```python
from build123d import *

# Parameters (mm, degrees)
F0_R     = 1.5
F1_DEPTH = 17
F2_DEPTH = 2
F3_R     = 5


with BuildPart() as f1:
    # F0 (on Top) → F1 (new body)
    with BuildSketch(Plane.XY):
        with BuildLine():
            ThreePointArc((21.4336734694, 1.6874956615), (21.4834119682, 0.8443993155), (21.5, 0))
            ThreePointArc((21.5, 0), (21.4834119682, -0.8443993155), (21.4336734694, -1.6874956615))
            ThreePointArc((21.4336734694, -1.6874956615), (22.0184319463, -2.4681612579), (22.7959183673, -3.0571401324))
            ThreePointArc((22.7959183673, -3.0571401324), (22.9489228772, -1.531972185), (23, 0))
            ThreePointArc((23, 0), (22.9489228772, 1.531972185), (22.7959183673, 3.0571401324))
            ThreePointArc((22.7959183673, 3.0571401324), (22.0184319463, 2.4681612579), (21.4336734694, 1.6874956615))
        make_face()
        with BuildLine():
            ThreePointArc((-21.4336734694, 1.6874956615), (0, 21.5), (21.4336734694, 1.6874956615))
            ThreePointArc((21.4336734694, 1.6874956615), (22.0184319463, 2.4681612579), (22.7959183673, 3.0571401324))
            ThreePointArc((22.7959183673, 3.0571401324), (0, 23), (-22.7959183673, 3.0571401324))
            ThreePointArc((-22.7959183673, 3.0571401324), (-22.0184319463, 2.4681612579), (-21.4336734694, 1.6874956615))
        make_face()
        with BuildLine():
            ThreePointArc((22.7959183673, -3.0571401324), (22.0184319463, -2.4681612579), (21.4336734694, -1.6874956615))
            ThreePointArc((21.4336734694, -1.6874956615), (0, -21.5), (-21.4336734694, -1.6874956615))
            ThreePointArc((-21.4336734694, -1.6874956615), (-22.0184319463, -2.4681612579), (-22.7959183673, -3.0571401324))
            ThreePointArc((-22.7959183673, -3.0571401324), (0, -23), (22.7959183673, -3.0571401324))
        make_face()
        with BuildLine():
            ThreePointArc((-21.4336734694, -1.6874956615), (-21.5, 0), (-21.4336734694, 1.6874956615))
            ThreePointArc((-21.4336734694, 1.6874956615), (-22.0184319463, 2.4681612579), (-22.7959183673, 3.0571401324))
            ThreePointArc((-22.7959183673, 3.0571401324), (-22.9489228772, 1.531972185), (-23, 0))
            ThreePointArc((-23, 0), (-22.9489228772, -1.531972185), (-22.7959183673, -3.0571401324))
            ThreePointArc((-22.7959183673, -3.0571401324), (-22.0184319463, -2.4681612579), (-21.4336734694, -1.6874956615))
        make_face()
        with BuildLine():
            ThreePointArc((28, 0), (26.2728105209, 3.0178043106), (22.7959183673, 3.0571401324))
            ThreePointArc((22.7959183673, 3.0571401324), (22.9489228772, 1.531972185), (23, 0))
            ThreePointArc((23, 0), (22.9489228772, -1.531972185), (22.7959183673, -3.0571401324))
            ThreePointArc((22.7959183673, -3.0571401324), (26.2728105209, -3.0178043106), (28, 0))
        make_face()
        with BuildLine():
            ThreePointArc((26, 0), (24.5, -1.5), (23, 0))
            ThreePointArc((23, 0), (24.5, 1.5), (26, 0))
        make_face(mode=Mode.SUBTRACT)
        with BuildLine():
            ThreePointArc((-23, 0), (-22.9489228772, 1.531972185), (-22.7959183673, 3.0571401324))
            ThreePointArc((-22.7959183673, 3.0571401324), (-28, 0), (-22.7959183673, -3.0571401324))
            ThreePointArc((-22.7959183673, -3.0571401324), (-22.9489228772, -1.531972185), (-23, 0))
        make_face()
        with Locations((-24.5, 0)):
            Circle(F0_R, mode=Mode.SUBTRACT)
    extrude(amount=F1_DEPTH)

    # F0 (on Top) → F2 (join)
    with BuildSketch(Plane.XY):
        with BuildLine():
            ThreePointArc((21.4336734694, 1.6874956615), (21.4834119682, 0.8443993155), (21.5, 0))
            ThreePointArc((21.5, 0), (21.4834119682, -0.8443993155), (21.4336734694, -1.6874956615))
            ThreePointArc((21.4336734694, -1.6874956615), (22.0184319463, -2.4681612579), (22.7959183673, -3.0571401324))
            ThreePointArc((22.7959183673, -3.0571401324), (22.9489228772, -1.531972185), (23, 0))
            ThreePointArc((23, 0), (22.9489228772, 1.531972185), (22.7959183673, 3.0571401324))
            ThreePointArc((22.7959183673, 3.0571401324), (22.0184319463, 2.4681612579), (21.4336734694, 1.6874956615))
        make_face()
        with BuildLine():
            ThreePointArc((-21.4336734694, 1.6874956615), (0, 21.5), (21.4336734694, 1.6874956615))
            ThreePointArc((21.4336734694, 1.6874956615), (22.0184319463, 2.4681612579), (22.7959183673, 3.0571401324))
            ThreePointArc((22.7959183673, 3.0571401324), (0, 23), (-22.7959183673, 3.0571401324))
            ThreePointArc((-22.7959183673, 3.0571401324), (-22.0184319463, 2.4681612579), (-21.4336734694, 1.6874956615))
        make_face()
        with BuildLine():
            ThreePointArc((22.7959183673, -3.0571401324), (22.0184319463, -2.4681612579), (21.4336734694, -1.6874956615))
            ThreePointArc((21.4336734694, -1.6874956615), (0, -21.5), (-21.4336734694, -1.6874956615))
            ThreePointArc((-21.4336734694, -1.6874956615), (-22.0184319463, -2.4681612579), (-22.7959183673, -3.0571401324))
            ThreePointArc((-22.7959183673, -3.0571401324), (0, -23), (22.7959183673, -3.0571401324))
        make_face()
        with BuildLine():
            ThreePointArc((-21.4336734694, -1.6874956615), (-21.5, 0), (-21.4336734694, 1.6874956615))
            ThreePointArc((-21.4336734694, 1.6874956615), (-22.0184319463, 2.4681612579), (-22.7959183673, 3.0571401324))
            ThreePointArc((-22.7959183673, 3.0571401324), (-22.9489228772, 1.531972185), (-23, 0))
            ThreePointArc((-23, 0), (-22.9489228772, -1.531972185), (-22.7959183673, -3.0571401324))
            ThreePointArc((-22.7959183673, -3.0571401324), (-22.0184319463, -2.4681612579), (-21.4336734694, -1.6874956615))
        make_face()
        with BuildLine():
            ThreePointArc((28, 0), (26.2728105209, 3.0178043106), (22.7959183673, 3.0571401324))
            ThreePointArc((22.7959183673, 3.0571401324), (22.9489228772, 1.531972185), (23, 0))
            ThreePointArc((23, 0), (22.9489228772, -1.531972185), (22.7959183673, -3.0571401324))
            ThreePointArc((22.7959183673, -3.0571401324), (26.2728105209, -3.0178043106), (28, 0))
        make_face()
        with BuildLine():
            ThreePointArc((26, 0), (24.5, -1.5), (23, 0))
            ThreePointArc((23, 0), (24.5, 1.5), (26, 0))
        make_face(mode=Mode.SUBTRACT)
        with BuildLine():
            ThreePointArc((-23, 0), (-22.9489228772, 1.531972185), (-22.7959183673, 3.0571401324))
            ThreePointArc((-22.7959183673, 3.0571401324), (-28, 0), (-22.7959183673, -3.0571401324))
            ThreePointArc((-22.7959183673, -3.0571401324), (-22.9489228772, -1.531972185), (-23, 0))
        make_face()
        with Locations((-24.5, 0)):
            Circle(F0_R, mode=Mode.SUBTRACT)
        with BuildLine():
            ThreePointArc((21.4336734694, -1.6874956615), (21, 0), (21.4336734694, 1.6874956615))
            ThreePointArc((21.4336734694, 1.6874956615), (0, 21.5), (-21.4336734694, 1.6874956615))
            ThreePointArc((-21.4336734694, 1.6874956615), (-21.1101517101, 0.8711650655), (-21, 0))
            ThreePointArc((-21, 0), (-21.1101517101, -0.8711650655), (-21.4336734694, -1.6874956615))
            ThreePointArc((-21.4336734694, -1.6874956615), (0, -21.5), (21.4336734694, -1.6874956615))
        make_face()
        with BuildLine():
            ThreePointArc((-21, 0), (-21.1101517101, 0.8711650655), (-21.4336734694, 1.6874956615))
            ThreePointArc((-21.4336734694, 1.6874956615), (-21.5, 0), (-21.4336734694, -1.6874956615))
            ThreePointArc((-21.4336734694, -1.6874956615), (-21.1101517101, -0.8711650655), (-21, 0))
        make_face()
        with BuildLine():
            ThreePointArc((21.4336734694, -1.6874956615), (21.4834119682, -0.8443993155), (21.5, 0))
            ThreePointArc((21.5, 0), (21.4834119682, 0.8443993155), (21.4336734694, 1.6874956615))
            ThreePointArc((21.4336734694, 1.6874956615), (21, 0), (21.4336734694, -1.6874956615))
        make_face()
        with Locations((-24.5, 0)):
            Circle(F0_R)
        with BuildLine():
            ThreePointArc((26, 0), (24.5, 1.5), (23, 0))
            ThreePointArc((23, 0), (24.5, -1.5), (26, 0))
        make_face()
    extrude(amount=F2_DEPTH)

    # F3
    f3_edges = [f1.edges().sort_by_distance(p)[0] for p in [
        (-22.795918, 3.05714, 8.5),
        (-22.795918, -3.05714, 8.5),
        (22.795918, -3.05714, 8.5),
        (22.795918, 3.05714, 8.5),
    ]]
    fillet(f3_edges, radius=F3_R)


solid = f1.part
```
Part model, mm, in its own coordinate system. A direction names the side the tool comes from. Give positions to 0.01 mm unless a question says otherwise; leave off trailing zeros. Write each loop counter-clockwise with the first axis right and the second up, starting at its lowest first coordinate (ties: lowest second). Pieces come first, ordered by that corner, then holes. Notation, with made-up numbers: (-4, 26.5) -> (21, 26.5) arc R29 ccw to (21, 50.5) -> close; hole circle Ø6 at (64.5, -2). An arc over 180 degrees is marked (long way). Put each result on its own line as item: value. Start each with the question number.
Item 1: Pull direction X, two halves, no side cores. Call faces 1 (the face through (0, 0, 0)), 2 (the face through (24, 0, 2)), 3 (the face through (0, -23, 8)): pulls with the +X half, pulls with the -X half, needs draft (parallel to the pull), parting line crosses it, or undercut.
Item 2: Cut at B-B (y = 10.5). List the corners of the cut face in (x, z), then the cut area to 3 significant figures.
Item 3: Which spindle directions (+Z, -Z, +X, -X, +Y, -Y) get a long thin tool onto all of the face, cutting with end or side? Do faces 4 (the face through (0, 0, 2)), 5 (the face through (0, 23, 8)). Say none if no direction does.
Item 4: Cut at A-A (x = 7.5). List the corners of the cut face in (y, z).
Item 5: Pin check, flat tips, straight feed: pin 1 Ø1.5 at (x, y) = (-25, 0) entering from +Z; pin 2 Ø6 at (y, z) = (13.5, 5.5) entering from -X; pin 3 Ø6 at (y, z) = (11, 9) entering from +X; pin 4 Ø3.5 at (x, y) = (25, -0.5) entering from +Z. Stop position of each tip, or through.
Item 6: Wall check: L1, parallel to Z at x = 15, y = -1; L2, parallel to X at y = 2, z = 3.25; L3, parallel to Y at x = -24.5, z = 6. Give the ranges that are in metal, low to high. Write a range as [from, to].
Answer list:
1. face 1: needs draft
1. face 2: undercut
1. face 3: parting line crosses it
2. outline: (-20.46, 0) -> (20.46, 0) -> (20.46, 17) -> (18.76, 17) -> (18.76, 2) -> (-18.76, 2) -> (-18.76, 17) -> (-20.46, 17) -> close
2. area: 133 mm2
3. face 4: +Z
3. face 5: +Z, -Z, +Y
4. outline: (-21.74, 0) -> (21.74, 0) -> (21.74, 17) -> (20.15, 17) -> (20.15, 2) -> (-20.15, 2) -> (-20.15, 17) -> (-21.74, 17) -> close
5. pin 1: stops at z = 2
5. pin 2: stops at x = -20.46
5. pin 3: stops at x = 21.56
5. pin 4: stops at z = 17
6. L1: z = [0, 2]
6. L2: x = [-27.37, -21.41], [21.41, 27.37]
6. L3: y = [-3.74, -1.5], [1.5, 3.74]
